CAD build for the part. Positions are in the model's coordinates, mm. Give positions to 0.01 mm unless a question says otherwise; leave off trailing zeros. Loops run counter-clockwise (first coordinate to the right, second up) from the corner with the lowest first, then second, coordinate; pieces in that order, holes last. Notation, with made-up numbers: (75, -0.5) -> (88, -0.5) arc R16 ccw to (88, 27.5) -> close; hole circle Ø6 at (-21.5, 26.5). An arc over 180 degrees is marked (long way). Write each question's results on one line, items separated by ' | '. Start each with the question number.
```python
from build123d import *

# Parameters (mm, degrees)
F0_R     = 10
F1_DEPTH = 110
F3_R     = 10
F3_R_2   = 9.5
F4_DEPTH = 1.3
F6_R     = 10
F6_R_2   = 9.5
F7_DEPTH = 1.3
F8_SIZE  = 0.5


with BuildPart() as f1:
    # F0 (on Front) → F1 (new body)
    with BuildSketch(Plane.XZ):
        Circle(F0_R)
    extrude(amount=F1_DEPTH)

    # F3 (on offset) → F4 (cut)
    with BuildSketch(Plane.XZ.offset(108)):
        Circle(F3_R)
        Circle(F3_R_2, mode=Mode.SUBTRACT)
    extrude(amount=-F4_DEPTH, mode=Mode.SUBTRACT)

    # F6 (on offset) → F7 (cut)
    with BuildSketch(Plane(origin=(0, -2, 0), x_dir=(1, 0, 0), z_dir=(0, 1, 0))):
        Circle(F6_R)
        Circle(F6_R_2, mode=Mode.SUBTRACT)
    extrude(amount=-F7_DEPTH, mode=Mode.SUBTRACT)

    # F8
    f8_edges = [f1.edges().sort_by_distance(p)[0] for p in [
        (-10, -110, 0),
        (-10, 0, 0),
    ]]
    chamfer(f8_edges, length=F8_SIZE)


solid = f1.part
```
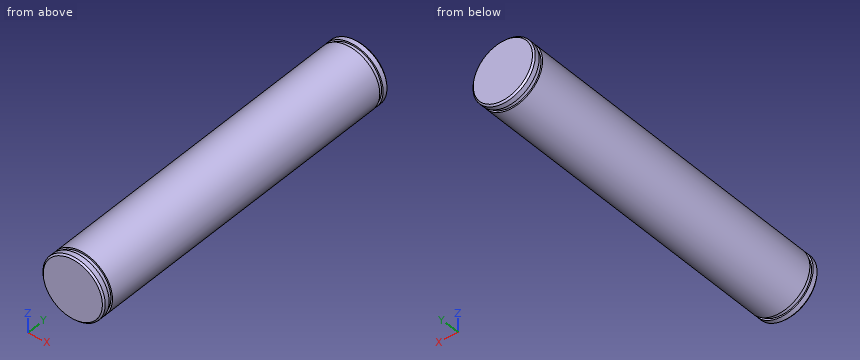
Q1. Saw through at A-A, the plane y = -72. List the corners of the cut face in (x, z).
Q2. Wall check: L1, parallel to Y at x = 7, z = -6.5; L2, parallel to Z at x = 0, y = -6; L3, parallel to Z at x = -7.75, y = -47. Give the ranges that are in metal, low to high.
Q3. Drop flat-ended pins along their axis: pin 1 (4 mm diameter, centred on y = -43.5, z = 3, fed in from +X); pin 2 (10 mm diameter, centred on y = -21, z = 7.5, fed in from -X); pin 3 (1 mm diameter, centred on y = -70, z = -7.5, fed in from -X). Give the stop position or say it passes through.
Answer block:
1) outline: circle Ø20 at (0, 0)
2) L1: y = -109.95 to -108, -106.7 to -3.3, -2 to -0.05 | L2: z = -10 to 10 | L3: z = -6.32 to 6.32
3) pin 1: stops at x = 9.95 | pin 2: stops at x = -9.68 | pin 3: stops at x = -7.14
